Check sheet for the modelled part. Datum: model origin and axes. Units: mm. Face numbers are marked on the shaded views. A direction names the side the tool comes from. Round coordinates to 2 decimals unless told otherwise and drop trailing zeros. Order: outer loops, then holes, each group sorted by start corner. A loop starts at its lowest first (then second) coordinate and runs counter-clockwise, first axis right, second up. Notation, with made-up numbers: (1, 47.25) -> (34, 47.25) arc R33 ccw to (34, 78.25) -> close; hole circle Ø2 at (-12, -13). An arc over 180 degrees is marked (long way). Answer in a Markdown table with one row per item.
from build123d import *

# Parameters (mm, degrees)
BOSS_EXTRUDE1_DEPTH = 40
SHELL1_T            = -1


with BuildPart() as part:
    # Sketch1 → Boss-Extrude1 (new body)
    with BuildSketch(Plane(origin=(0, 0, 0), x_dir=(1, 0, 0), z_dir=(0, 1, 0))):
        with BuildLine():
            Line((-45, 0), (-45, -50))
            Line((-45, -50), (45, -50))
            Line((45, -50), (45, 0))
            ThreePointArc((45, 0), (0, 45), (-45, 0))
        make_face()
    extrude(amount=BOSS_EXTRUDE1_DEPTH)

    # Shell1
    shell1_openings = [part.faces().sort_by_distance(p)[0] for p in [
        (0, 40, 13.75),
    ]]
    offset(amount=SHELL1_T, openings=shell1_openings, kind=Kind.INTERSECTION)


solid = part.part
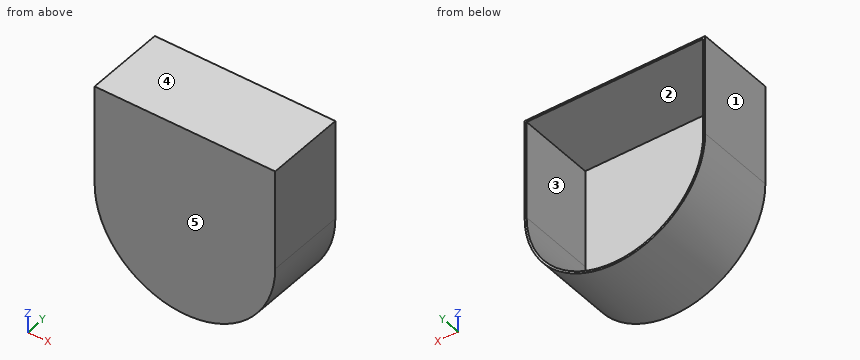
Item 1: Mould release check, pull along Z, two halves, no side actions. Record for the marked faces 3, 4 and 5: pulls with the +Z half, pulls with the -Z half, needs draft (parallel to the pull), parting line crosses it, or undercut.
Result sheet:
| item | result |
|---|---|
| face 3 | undercut |
| face 4 | pulls with the +Z half |
| face 5 | needs draft |
Item 2: Set-up check for the marked faces 1 and 2: record each of +Z, -Z, +X, -X, +Y, -Y from which the full face is reachable in a straight line by a thin tool's end or side.
Result sheet:
| item | result |
|---|---|
| face 1 | +Z, -Z, -X, +Y, -Y |
| face 2 | +Y |
Item 3: Depth check by flat-ended pin: P1, Ø6, axis at x = 0.5, z = -34.5, coming from the +Y side; P2, Ø1, axis at y = 15, z = -23, coming from the +X side; P3, Ø1, axis at y = 15, z = -33, coming from the -X side. Enter the tip coordinate at first touch or a pass-through.
Result sheet:
| item | result |
|---|---|
| P1 | stops at y = 1 |
| P2 | stops at x = 38.97 |
| P3 | stops at x = -31.12 |
Item 4: Cross-section at B-B (x = 0). Record the boundary of the cut face in (y, z), and give its area (3 significant figures).
Result sheet:
| item | result |
|---|---|
| outline | (0, -45) -> (40, -45) -> (40, -44) -> (1, -44) -> (1, 49) -> (40, 49) -> (40, 50) -> (0, 50) -> close |
| area | 173 mm^2 |
Item 5: Cross-section at A-A (y = 16). Record the boundary of the cut face in (x, z).
Result sheet:
| item | result |
|---|---|
| outline | (-45, 0) arc R45 ccw to (45, 0) -> (45, 50) -> (-45, 50) -> close; hole (-44, 0) arc R44 ccw to (44, 0) -> (44, 49) -> (-44, 49) -> close |
Item 6: Scan lines: line 1 (X direction, y = 9, z = 26); line 2 (Y direction, x = 18.5, z = -16); line 3 (Z direction, x = -9, y = 29). Record each from-to range of solid material in increasing order. Write a range as [from, to].
Result sheet:
| item | result |
|---|---|
| line 1 | x = [-45, -44], [44, 45] |
| line 2 | y = [0, 1] |
| line 3 | z = [-44.09, -43.07], [49, 50] |
Item 7: Cross-section at C-C (z = -25). Record the boundary of the cut face in (x, y).
Result sheet:
| item | result |
|---|---|
| outline | (-37.42, 0) -> (37.42, 0) -> (37.42, 40) -> (36.21, 40) -> (36.21, 1) -> (-36.21, 1) -> (-36.21, 40) -> (-37.42, 40) -> close |
